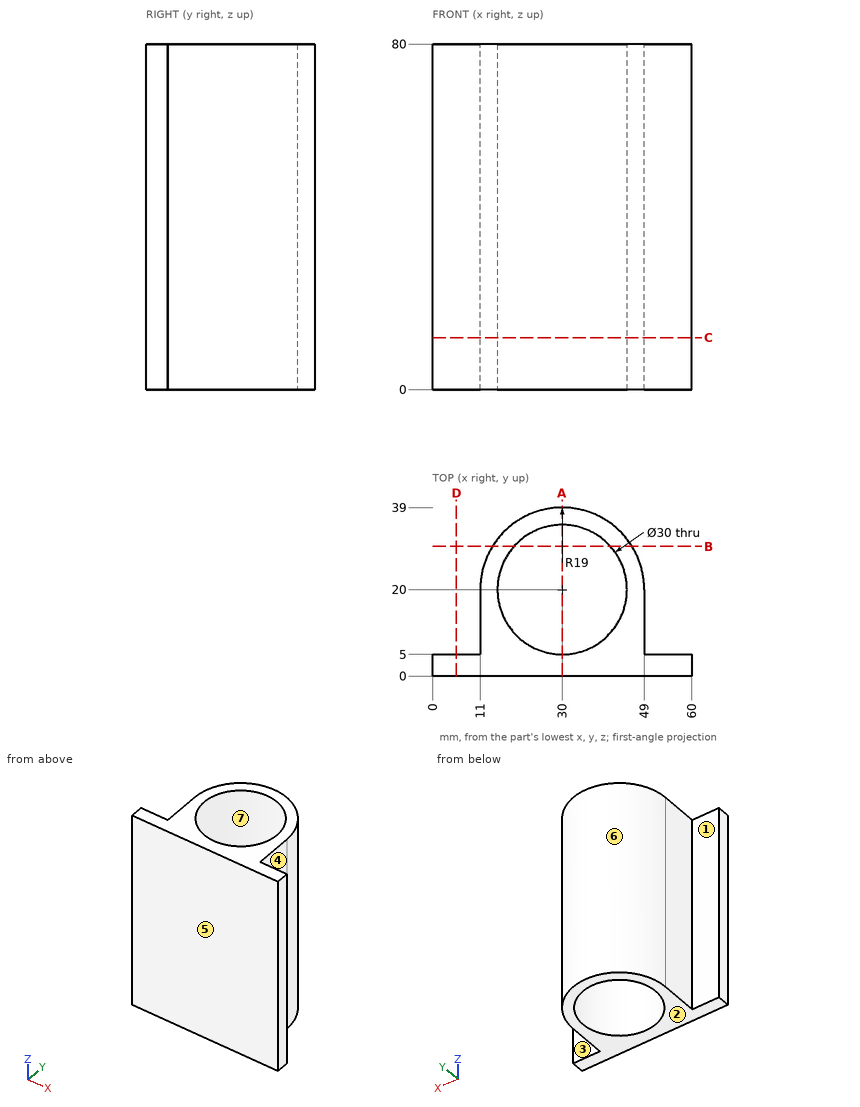
Print and shaded views of the part. All mm, measured from the part's lowest x, y and z. A direction names the side the tool comes from. Round coordinates to 2 decimals unless told otherwise and drop trailing zeros. Loops run counter-clockwise (first coordinate to the right, second up) from the corner with the lowest first, then second, coordinate; pieces in that order, holes last. Notation, with made-up numbers: (5.5, -7) -> (9.5, -7) arc R24 ccw to (9.5, 7) -> close; hole circle Ø4 at (44.25, 71). An arc over 180 degrees is marked (long way). Use CSV: the item, a comma, the result in double quotes. Start each with the question number.
1) Wall check: L1, parallel to Y at x = 30, z = 51.5; L2, parallel to X at y = 6.5, z = 20; L3, parallel to Y at x = 7.5, z = 8.5. Give the ranges that are in metal, low to high. Write a range as [from, to].
2) Cut at A-A, the plane x = 30. Write the cut outline in (y, z), plus the area to 3 significant figures.
3) Cut at B-B, the plane y = 30. Write the cut outline in (x, z), plus the area to 3 significant figures.
4) Cut at C-C, the plane z = 12. Write the cut outline in (x, y).
5) Pull direction Y, two halves, no side cores. Call the marked faces 4, 5, 6 and 7: +Y half, -Y half, draft (parallel to the pull), parting line (faces both ways), or undercut.
6) Cut at D-D, the plane x = 5.5. Write the cut outline in (y, z), plus the area to 3 significant figures.
7) Drop flat-ended pins along their axis: P1, Ø12, axis at x = 52.5, y = 9, coming from the +Z side; P2, Ø6, axis at y = 26, z = 26.5, coming from the +X side; P3, Ø2, axis at y = 34.5, z = 27, coming from the -X side; P4, Ø16.5, axis at y = 15, z = 49, coming from the +X side. Give the stop position or say it passes through.
8) Which spindle directions (+Z, -Z, +X, -X, +Y, -Y) get a long thin tool onto all of the face, cutting with end or side? Do the marked faces 1, 2 and 3. Say none if no direction does.
Determined:
1,L1,"y = [0, 5], [35, 39]"
1,L2,"x = [11, 23.46], [36.54, 49]"
1,L3,"y = [0, 5]"
2,outline,"(0, 0) -> (5, 0) -> (5, 80) -> (0, 80) -> close; (35, 0) -> (39, 0) -> (39, 80) -> (35, 80) -> close"
2,area,"720 mm2"
3,outline,"(13.84, 0) -> (18.82, 0) -> (18.82, 80) -> (13.84, 80) -> close; (41.18, 0) -> (46.16, 0) -> (46.16, 80) -> (41.18, 80) -> close"
3,area,"796 mm2"
4,outline,"(0, 0) -> (60, 0) -> (60, 5) -> (49, 5) -> (49, 20) arc R19 ccw to (11, 20) -> (11, 5) -> (0, 5) -> close; hole circle Ø30 at (30, 20)"
5,face 4,"draft"
5,face 5,"-Y half"
5,face 6,"+Y half"
5,face 7,"undercut"
6,outline,"(0, 0) -> (5, 0) -> (5, 80) -> (0, 80) -> close"
6,area,"400 mm2"
7,P1,"stops at z = 80"
7,P2,"stops at x = 48.76"
7,P3,"stops at x = 16.63"
7,P4,"stops at x = 49"
8,face 1,"+Z, -Z, -X, +Y"
8,face 2,"-Z, +X, -X, +Y, -Y"
8,face 3,"+Z, -Z, +X, +Y"
